from build123d import *

# Parameters (mm, degrees)
BOSS_EXTRUDE1_DEPTH = 23
BOSS_EXTRUDE3_DEPTH = 2
SKETCH4_W           = 20
SKETCH4_H           = 41
CUT_EXTRUDE1_DEPTH  = 18.2
SKETCH5_R           = 10
SKETCH5_R_2         = 4.25
BOSS_EXTRUDE4_DEPTH = 0.7
CUT_EXTRUDE2_REACH  = 80.949
SKETCH6_R           = 1.05
SKETCH6_R_2         = 4.25
BOSS_EXTRUDE5_START = 6.1
SKETCH7_R           = 10
BOSS_EXTRUDE5_DEPTH = 6.1
SKETCH11_R          = 4
BOSS_EXTRUDE6_DEPTH = 0.5
SKETCH10_R          = 3
CUT_EXTRUDE4_DEPTH  = 7.2
CUT_EXTRUDE3_REACH  = 80.949
SKETCH9_R           = 1.475
SKETCH12_R          = 5
CUT_EXTRUDE5_DEPTH  = 4
SKETCH13_R          = 10
SKETCH13_R_2        = 4
CUT_EXTRUDE6_DEPTH  = 3.5
FILLET2_R           = 2


with BuildPart() as part:
    # Sketch1 → Boss-Extrude1 (new, symmetric)
    with BuildSketch(Plane.XY):
        with BuildLine():
            Line((0, 59.9), (16.889174661, 50.149030463))
            ThreePointArc((16.889174661, 50.149030463), (17.524957173, 29.799404984), (0, 19.43661807))
            Line((0, 19.43661807), (0, 10))
            ThreePointArc((0, 10), (-3.934485272, -9.193466465), (7.234311682, 6.903965128))
            Line((7.234311682, 6.903965128), (7.234311682, 17.603965128))
            ThreePointArc((7.234311682, 17.603965128), (22.931748607, 37.666051544), (10.5, 59.9))
            Line((10.5, 59.9), (0, 59.9))
        make_face()
    extrude(amount=BOSS_EXTRUDE1_DEPTH, both=True)

    # Sketch3 → Boss-Extrude3 (add)
    with BuildSketch(Plane.XY.offset(23)):
        with BuildLine():
            Line((0, 59.9), (0, 19.43661807))
            ThreePointArc((0, 19.43661807), (17.524957173, 29.799404984), (16.889174661, 50.149030463))
            Line((16.889174661, 50.149030463), (0, 59.9))
        make_face()
    boss_extrude3 = extrude(amount=-BOSS_EXTRUDE3_DEPTH)

    # Mirror1: Boss-Extrude3 across plane
    add(boss_extrude3.mirror(Plane.XY))

    # Sketch4 → Cut-Extrude1 (cut, symmetric)
    with BuildSketch(Plane(origin=(0, 0, 0), x_dir=(1, 0, 0), z_dir=(0, 1, 0))):
        Rectangle(SKETCH4_W, SKETCH4_H)
    extrude(amount=CUT_EXTRUDE1_DEPTH, both=True, mode=Mode.SUBTRACT)

    # Sketch5 → Boss-Extrude4 (add)
    with BuildSketch(Plane(origin=(0, 0, 20.5), x_dir=(-1, 0, 0), z_dir=(0, 0, -1))):
        Circle(SKETCH5_R)
        Circle(SKETCH5_R_2, mode=Mode.SUBTRACT)
    extrude(amount=BOSS_EXTRUDE4_DEPTH)

    # Sketch6 → Cut-Extrude2 (cut, up to next)
    with BuildSketch(Plane.XY.offset(23), mode=Mode.PRIVATE) as cut_extrude2_sk1:
        with Locations((0, 7)):
            Circle(SKETCH6_R)
    cut_extrude2_tool1 = extrude(cut_extrude2_sk1.sketch, amount=-CUT_EXTRUDE2_REACH, mode=Mode.PRIVATE) & part.part
    # Sketch6 → Cut-Extrude2 (cut, up to next)
    with BuildSketch(Plane.XY.offset(23), mode=Mode.PRIVATE) as cut_extrude2_sk2:
        with Locations((7, 0)):
            Circle(SKETCH6_R)
    cut_extrude2_tool2 = extrude(cut_extrude2_sk2.sketch, amount=-CUT_EXTRUDE2_REACH, mode=Mode.PRIVATE) & part.part
    # Sketch6 → Cut-Extrude2 (cut, up to next)
    with BuildSketch(Plane.XY.offset(23), mode=Mode.PRIVATE) as cut_extrude2_sk3:
        with Locations((0, -7)):
            Circle(SKETCH6_R)
    cut_extrude2_tool3 = extrude(cut_extrude2_sk3.sketch, amount=-CUT_EXTRUDE2_REACH, mode=Mode.PRIVATE) & part.part
    # Sketch6 → Cut-Extrude2 (cut, up to next)
    with BuildSketch(Plane.XY.offset(23), mode=Mode.PRIVATE) as cut_extrude2_sk4:
        with Locations((-7, 0)):
            Circle(SKETCH6_R)
    cut_extrude2_tool4 = extrude(cut_extrude2_sk4.sketch, amount=-CUT_EXTRUDE2_REACH, mode=Mode.PRIVATE) & part.part
    # Sketch6 → Cut-Extrude2 (cut, up to next)
    with BuildSketch(Plane.XY.offset(23), mode=Mode.PRIVATE) as cut_extrude2_sk5:
        Circle(SKETCH6_R_2)
    cut_extrude2_tool5 = extrude(cut_extrude2_sk5.sketch, amount=-CUT_EXTRUDE2_REACH, mode=Mode.PRIVATE) & part.part
    add(cut_extrude2_tool1.solids().sort_by_distance((0, 7, 23))[0], mode=Mode.SUBTRACT)
    add(cut_extrude2_tool2.solids().sort_by_distance((7, 0, 23))[0], mode=Mode.SUBTRACT)
    add(cut_extrude2_tool3.solids().sort_by_distance((0, -7, 23))[0], mode=Mode.SUBTRACT)
    add(cut_extrude2_tool4.solids().sort_by_distance((-7, 0, 23))[0], mode=Mode.SUBTRACT)
    add(cut_extrude2_tool5.solids().sort_by_distance((0, 0, 23))[0], mode=Mode.SUBTRACT)

    # Sketch7 → Boss-Extrude5 (add)
    with BuildSketch(Plane.XY.offset(-20.5).offset(BOSS_EXTRUDE5_START)):
        with Locations(Location((0, 0, 0), (0, 0, 90))):
            Circle(SKETCH7_R)
    extrude(amount=-BOSS_EXTRUDE5_DEPTH)

    # Sketch11 → Boss-Extrude6 (add)
    with BuildSketch(Plane.XY.offset(-14.4)):
        Circle(SKETCH11_R)
    extrude(amount=BOSS_EXTRUDE6_DEPTH)

    # Sketch10 → Cut-Extrude4 (cut)
    with BuildSketch(Plane(origin=(0, 0, -23), x_dir=(-1, 0, 0), z_dir=(0, 0, -1))):
        Circle(SKETCH10_R)
    extrude(amount=-CUT_EXTRUDE4_DEPTH, mode=Mode.SUBTRACT)

    # Sketch9 → Cut-Extrude3 (cut, up to next)
    with BuildSketch(Plane(origin=(0, 0, -23), x_dir=(-1, 0, 0), z_dir=(0, 0, -1)), mode=Mode.PRIVATE) as cut_extrude3_sk1:
        Circle(SKETCH9_R)
    cut_extrude3_tool1 = extrude(cut_extrude3_sk1.sketch, amount=-CUT_EXTRUDE3_REACH, mode=Mode.PRIVATE) & part.part
    add(cut_extrude3_tool1.solids().sort_by_distance((0, 0, -23))[0], mode=Mode.SUBTRACT)

    # Sketch12 → Cut-Extrude5 (cut)
    with BuildSketch(Plane(origin=(0, 0, -23), x_dir=(-1, 0, 0), z_dir=(0, 0, -1))):
        Circle(SKETCH12_R)
    extrude(amount=-CUT_EXTRUDE5_DEPTH, mode=Mode.SUBTRACT)

    # Sketch13 → Cut-Extrude6 (cut)
    with BuildSketch(Plane.XY.offset(-14.4)):
        with Locations(Location((0, 0, 0), (0, 0, 90))):
            Circle(SKETCH13_R)
        Circle(SKETCH13_R_2, mode=Mode.SUBTRACT)
    extrude(amount=-CUT_EXTRUDE6_DEPTH, mode=Mode.SUBTRACT)

    # Fillet2
    fillet2_edges = [part.edges().sort_by_distance(p)[0] for p in [
        (-4, 0, -17.9),
    ]]
    fillet(fillet2_edges, radius=FILLET2_R)


solid = part.part
Source: CAD feature listing. Evaluate the final solid. Frame: model axes, mm. A direction names the side the tool comes from. Round coordinates to 2 decimals unless told otherwise and drop trailing zeros. Loops run counter-clockwise (first coordinate to the right, second up) from the corner with the lowest first, then second, coordinate; pieces in that order, holes last. Notation, with made-up numbers: M 70,23 L 117,23 A6 cw 117,31 Z; hole C 36,3.25 d4. An arc over 180 degrees is marked long. Return JSON: item names as keys, results as strings. Group by question number.
1. Mould query, pull axis Z, two halves, no side actions, for faces 6 (the face through (3, 0, -17)), 7 (the face through (3, 14, -20.5)), 8 (the face through (6, 25, 23)). Classes: released by +Z, released by -Z, zero draft, split by the parting line, or undercut.
2. Pin query (flat end, axial travel): pin 1 (1.7 mm diameter, centred on x = -7, y = 0, fed in from +Z); pin 2 (7.5 mm diameter, centred on x = 0, y = 0, fed in from +Z); pin 3 (1.2 mm diameter, centred on y = 13, z = 21, fed in from +X). Return the tip coordinate at first contact, or that it passes through.
3. Section query A-A on y = -7. Output: boundary loops of the cut face in (x, z).
4. Section query C-C on z = 9. Output: boundary loops of the cut face in (x, y).
5. Material intervals for line 1 along Z through (x, y) = (7, 15); line 2 along Z through (x, y) = (11, 36); line 3 along Y through (x, z) = (9, -20), sorted ascending. Write a range as from..to.
6. Section query D-D on y = 42. Output: boundary loops of the cut face in (x, z), and give its area (3 significant figures).
7. Reachability of faces 1 (the face through (2, 0, -13.9)), 2 (the face through (7.234, 12, 22)), 3 (the face through (1.08, -4.88, -21.03)), 4 (the face through (8.33, 55.09, 0.29)), 5 (the face through (-1.05, 7.05, 21.42)) from +Z, -Z, +X, -X, +Y, -Y: full face, straight path, thin tool, end or side. Return the list, or none.
Checks:
{
 "1": {"face 6": "zero draft", "face 7": "undercut", "face 8": "released by +Z"},
 "2": {"pin 1": "stops at z = -17.9", "pin 2": "stops at z = -13.9", "pin 3": "stops at x = 7.23"},
 "3": {"outline": "M -7.14,-23 L 7.14,-23 L 7.14,-17.9 L -7.14,-17.9 Z; M -7.14,19.8 L -1.05,19.8 L -1.05,23 L -7.14,23 Z; M 1.05,19.8 L 7.14,19.8 L 7.14,23 L 1.05,23 Z"},
 "4": {"outline": "M 0,18.2 L 8.83,18.2 A23 ccw 10.5,59.9 L 0,59.9 L 16.89,50.15 A20 cw 0,19.44 Z"},
 "5": {"line 1": "z = -23..-20.5, 20.5..23", "line 2": "z = -23..-21, 21..23", "line 3": "y = -4.36..4.36, 18.27..21.58, 54.7..59.9"},
 "6": {"outline": "M 0,-23 L 22.86,-23 L 22.86,23 L 0,23 L 0,21 L 19.84,21 L 19.84,-21 L 0,-21 Z", "area": "218 mm²"},
 "7": {"face 1": "+Z, +X, -X, -Y", "face 2": "+Z, -Z, +X", "face 3": "-Z", "face 4": "-X", "face 5": "+Z"}
}
